Can you work these out from the model? Positions are in its coordinate system, mm. A direction names the side the tool comes from. Coordinates: 2 decimals unless noted, no trailing zeros. Loops run counter-clockwise (first coordinate to the right, second up) from the corner with the lowest first, then second, coordinate; pieces in that order, holes last.
Autodesk Inventor part; units mm, degrees
ref_plane "YZ Plane" through (0, 0, 0) normal (1, 0, 0) x (0, 1, 0)
ref_plane "XZ Plane" through (0, 0, 0) normal (0, 1, 0) x (-1, 0, 0)
ref_plane "XY Plane" through (0, 0, 0) normal (0, 0, 1) x (1, 0, 0)
sketch "Sketch1" plane through (0, 0, 0) normal (0, 1, 0) x (-1, 0, 0)
  circle A0 centre (0, 0) radius 36.71
  circle A1 centre (0, 0) radius 12.25
  dimension "d0" = 73.42
  dimension "d1" = 24.5
extrude "Extrusion1" add sketch "Sketch1" along normal blind 5.2
sketch "Sketch2" plane through (0, 0, 0) normal (0, -1, 0) x (1, 0, 0)
  circle A0 centre (0, 0) radius 36.71
  circle A1 centre (0, 0) radius 36.71
extrude "Extrusion2" add sketch "Sketch2" along normal blind 3 draft 30
chamfer "Chamfer1" distance 0.8 angle 45 1 edges at (36.71, 5.2, 0)
sketch "Sketch3" plane through (0, 0, 0) normal (0, 1, 0) x (1, 0, 0)
  circle A0 centre (0, 0) radius 12.25
extrude "Extrusion3" cut sketch "Sketch3" against normal blind 3
properties part number "base"
Item 1: Suppose I cut it at B-B, the plane x = 0. Please give me the cut outline in (y, z), plus the area to 3 significant figures.
Results are:
outline: (-3, -38.44) - (0, -36.71) - (4.4, -36.71) - (5.2, -35.91) - (5.2, -12.25) - (-3, -12.25) - close; (-3, 12.25) - (5.2, 12.25) - (5.2, 35.91) - (4.4, 36.71) - (0, 36.71) - (-3, 38.44) - close
area: 406 mm2
Item 2: I'm going to push flat-ended pins straight in: P1, Ø1, axis at y = -1, z = 23.5, coming from the +X side; P2, Ø22, axis at x = 0, z = 0, coming from the -Y side. Where does each tip first touch, or does it pass through?
Results are:
P1: stops at x = 29.49
P2: passes through
Item 3: On a 3-axis mill with a long thin cutter (end or side, diameter ignored), from which of +Z, -Z, +X, -X, +Y, -Y can I reach the whole of each face in a straight line? I mean faces 1 (the face through (-15, 5.2, 1)), 2 (the face through (7.958, 2.169, 35.837)). Say none if no direction works.
Results are:
face 1: +Z, -Z, +X, -X, +Y
face 2: +Y
Item 4: Suppose I cut it at A-A, the plane z = 0. Please give me the cut outline in (x, y), plus the area to 3 significant figures.
Results are:
outline: (-38.44, -3) - (-12.25, -3) - (-12.25, 5.2) - (-35.91, 5.2) - (-36.71, 4.4) - (-36.71, 0) - close; (12.25, -3) - (38.44, -3) - (36.71, 0) - (36.71, 4.4) - (35.91, 5.2) - (12.25, 5.2) - close
area: 406 mm2
Item 5: I need wall thicknesses on line 1 along X through (y, z) = (1.2, 0); line 2 along X through (y, z) = (-0.6, 0). Which ranges of each line are inside material? Lowest first, please.
Results are:
line 1: x = -36.71 to -12.25, 12.25 to 36.71
line 2: x = -37.06 to -12.25, 12.25 to 37.06
